```python
from build123d import *

# Parameters (mm, degrees)
SKETCH4_R          = 7.5
CUT_EXTRUDE1_DEPTH = 179.440382209
CIRPATTERN1_COUNT  = 9
CHAMFER1_SIZE      = 0.5
FILLET2_R          = 1


with BuildPart() as part:
    # Sketch1 → Revolve1 (revolve)
    with BuildSketch(Plane.XY, mode=Mode.PRIVATE) as revolve1_sk:
        with BuildLine():
            Line((111.519334361, 58.850307256), (111.519334361, 40))
            Line((111.519334361, 40), (116.519334361, 40))
            Line((116.519334361, 40), (116.519334361, 55.750229717))
            ThreePointArc((116.519334361, 55.750229717), (117.787313388, 54.801644975), (119.019334361, 53.806804209))
            Line((119.019334361, 53.806804209), (119.019334361, 40))
            Line((119.019334361, 40), (124.019334361, 40))
            Line((124.019334361, 40), (124.019334361, 48.86))
            Line((124.019334361, 48.86), (134.019334361, 48.86))
            Line((134.019334361, 48.86), (134, 37.5))
            Line((134, 37.5), (154, 37.5))
            Line((154, 37.5), (154, 30))
            Line((154, 30), (54, 30))
            Line((54, 30), (54, 15))
            Line((54, 15), (0, 15))
            Line((0, 15), (0, 35))
            Line((0, 35), (10, 35))
            Line((10, 35), (10, 25))
            Line((10, 25), (17, 25))
            ThreePointArc((17, 25), (24.071067812, 27.928932188), (27, 35))
            Line((27, 35), (27, 43))
            Line((27, 43), (44.019334361, 48.86022678))
            Line((44.019334361, 48.86022678), (59.019334361, 48.86022678))
            Line((59.019334361, 48.86022678), (59.019334361, 40))
            Line((59.019334361, 40), (64.019334361, 40))
            Line((64.019334361, 40), (64.019334361, 53.806967156))
            ThreePointArc((64.019334361, 53.806967156), (65.251355628, 54.801796268), (66.519334361, 55.750369564))
            Line((66.519334361, 55.750369564), (66.519334361, 40))
            Line((66.519334361, 40), (71.519334361, 40))
            Line((71.519334361, 40), (71.519334361, 58.850409967))
            ThreePointArc((71.519334361, 58.850409967), (72.75942837, 59.480289713), (74.019334361, 60.069542238))
            Line((74.019334361, 60.069542238), (74.019334361, 40))
            Line((74.019334361, 40), (79.019334361, 40))
            Line((79.019334361, 40), (79.019334361, 61.944697773))
            ThreePointArc((79.019334361, 61.944697773), (80.26417648, 62.304323607), (81.519334361, 62.626101999))
            Line((81.519334361, 62.626101999), (81.519334361, 40))
            Line((81.519334361, 40), (86.519334361, 40))
            Line((86.519334361, 40), (86.519334361, 63.517648918))
            ThreePointArc((86.519334361, 63.517648918), (87.767721666, 63.64596551), (89.019334361, 63.737626161))
            Line((89.019334361, 63.737626161), (89.019334361, 40))
            Line((89.019334361, 40), (94.019334361, 40))
            Line((94.019334361, 40), (94.019334361, 63.737614791))
            ThreePointArc((94.019334361, 63.737614791), (95.27094714, 63.645948403), (96.519334361, 63.51762606))
            Line((96.519334361, 63.51762606), (96.519334361, 40))
            Line((96.519334361, 40), (101.519334361, 40))
            Line((101.519334361, 40), (101.519334361, 62.626055303))
            ThreePointArc((101.519334361, 62.626055303), (102.774492344, 62.304270611), (104.019334361, 61.94463843))
            Line((104.019334361, 61.94463843), (104.019334361, 40))
            Line((104.019334361, 40), (109.019334361, 40))
            Line((109.019334361, 40), (109.019334361, 60.069455171))
            ThreePointArc((109.019334361, 60.069455171), (110.279240504, 59.480194874), (111.519334361, 58.850307256))
        make_face()
    revolve(revolve1_sk.sketch.rotate(Axis((-113.765130781, 0, 0), (1, 0, 0)), 180), axis=Axis((-113.765130781, 0, 0), (1, 0, 0)))

    # Sketch4 → Cut-Extrude1 (cut, through all)
    with BuildSketch(Plane(origin=(0, 0, 0), x_dir=(1, 0, 0), z_dir=(0, 1, 0))):
        with Locations(Location((91.519334361, 0, 0), (0, 0, 180))):
            Circle(SKETCH4_R)
    extrude(amount=-CUT_EXTRUDE1_DEPTH, mode=Mode.SUBTRACT)

    # Sketch11 → 5.0 mm Dowel Holes3 (revolve, cut)
    with BuildSketch(Plane(origin=(27, 39, 0), x_dir=(0, 0, 1), z_dir=(0, 1, 0))):
        Polygon((0, 0), (0, 21.502151548), (2.5, 20), (2.5, 0.209774908), (2.75, 0), align=None)
    f_5_0_mm_dowel_holes3 = revolve(axis=Axis((20.65, 39, 0), (1, 0, 0)), mode=Mode.SUBTRACT)

    # CirPattern1: 5.0 mm Dowel Holes3 ×9 about axis
    cirpattern1_axis = Axis((0, 0, 0), (1, 0, 0))
    for i in range(1, CIRPATTERN1_COUNT):
        add(f_5_0_mm_dowel_holes3.rotate(cirpattern1_axis, i * 360 / CIRPATTERN1_COUNT), mode=Mode.SUBTRACT)

    # Chamfer1
    chamfer1_edges = [part.edges().sort_by_distance(p)[0] for p in [
        (154, 30, 0),
        (0, 15, 0),
    ]]
    chamfer(chamfer1_edges, length=CHAMFER1_SIZE)

    # Fillet2
    fillet2_edges = [part.edges().sort_by_distance(p)[0] for p in [
        (0, 15.5, 0),
        (0, 35, 0),
    ]]
    fillet(fillet2_edges, radius=FILLET2_R)


solid = part.part
```
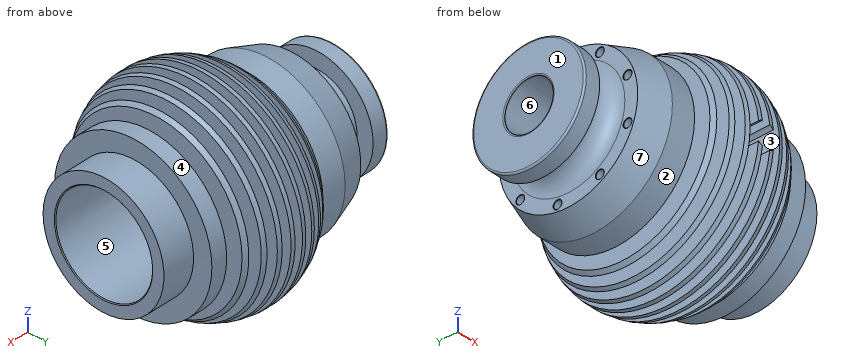
The model under review builds one solid part; all positions refer to its coordinate system, in mm. Face numbers are marked on the shaded views. A direction names the side the tool comes from. Round coordinates to 2 decimals unless told otherwise and drop trailing zeros. Order: outer loops, then holes, each group sorted by start corner. A loop starts at its lowest first (then second) coordinate and runs counter-clockwise, first axis right, second up. Notation, with made-up numbers: (-10.5, 34) -> (45.5, 34) arc R30 ccw to (45.5, 68) -> close; hole circle Ø8 at (-39, 16.5). An arc over 180 degrees is marked (long way). One line per item, written item: value. Start each with the question number.
Q1. Wall thickness on line 1 (X direction, y = 39, z = -48); line 2 (X direction, y = -32.5, z = 46); line 3 (Y direction, x = 32, z = -11.5): over which ranges is each line inside the solid? List them lowest first.
Q2. Machinability: for the marked faces 1, 2, 3 and 4, which of the approach directions +Z, -Z, +X, -X, +Y, -Y give a long, thin tool a straight path to every point of the face, cutting with its end or side? Answer none if there is none.
Q3. Clearance check with flat-ended pins moving along their axes: pin 1 Ø1 at (x, z) = (73, 49) entering from +Y; pin 2 Ø3 at (x, z) = (117, -23) entering from -Y; pin 3 Ø5 at (x, y) = (50, 27) entering from +Z. State where each tip first meets the part, or that it passes through.
Q4. Take a section at A-A (x = 15). Write out the cut boundary in (y, z).
Q5. Mouldability with a two-part tool opening along Y and no side actions: class the marked faces 5, 6 and 7 as released by +Y, released by -Y, zero draft, split by the parting line, or undercut.
Reported:
1. line 1: x = 79.02 to 81.52, 86.52 to 89.02, 94.02 to 96.52, 101.52 to 104.02
1. line 2: x = 71.52 to 74.02, 79.02 to 81.52, 86.52 to 89.02, 94.02 to 96.52, 101.52 to 104.02, 109.02 to 111.52
1. line 3: y = -43.22 to -38.34, -34.95 to -9.63, 9.63 to 43.22
2. face 1: +Z, -Z, -X, +Y, -Y
2. face 2: -X
2. face 3: none
2. face 4: +X
3. pin 1: stops at y = 34.74
3. pin 2: stops at y = -51.4
3. pin 3: stops at z = 42.27
4. outline: circle Ø50 at (0, 0); hole circle Ø30 at (0, 0)
5. face 5: undercut
5. face 6: undercut
5. face 7: split by the parting line
